```python
from build123d import *

# Parameters (mm, degrees)
EXTRUDE_1_DEPTH = 4
CHAMFER_1_SIZE  = 10


with BuildPart() as part:
    # Эскиз1 → Бобышка-Вытянуть1 (new, symmetric)
    with BuildSketch(Plane.XY):
        Polygon((0, 0), (0, 80), (8, 80), (70, 8), (70, 0), align=None)
    extrude(amount=EXTRUDE_1_DEPTH, both=True)

    # Фаска1
    chamfer_1_edges = [part.edges().sort_by_distance(p)[0] for p in [
        (0, 0, 0),
    ]]
    chamfer(chamfer_1_edges, length=CHAMFER_1_SIZE)


solid = part.part
```
Here's how the part is built. I have some questions about the finished solid (model axes, mm). Coordinates: 2 decimals unless noted, no trailing zeros. Loops run counter-clockwise (first coordinate to the right, second up) from the corner with the lowest first, then second, coordinate; pieces in that order, holes last. Notation, with made-up numbers: (11.25, -3) -> (31.25, -3) arc R21 cw to (31.25, 6) -> close; hole circle Ø8 at (-13, -12.5). An arc over 180 degrees is marked (long way). Return JSON: item names as keys, results as strings.
1) If we section it at C-C, the plane x = 45: Write out the boundary of the cut face in (y, z).
Results below:
{"outline": "(0, -4) -> (37.03, -4) -> (37.03, 4) -> (0, 4) -> close"}
2) If we section it at A-A, the plane z = -2: Write out the boundary of the cut face in (x, y).
Results below:
{"outline": "(0, 10) -> (10, 0) -> (70, 0) -> (70, 8) -> (8, 80) -> (0, 80) -> close"}
3) If we section it at B-B, the plane y = 41: Write out the boundary of the cut face in (x, z), then the cut area to 3 significant figures.
Results below:
{"outline": "(0, -4) -> (41.58, -4) -> (41.58, 4) -> (0, 4) -> close", "area": "333 mm²"}
4) I need wall thicknesses on line 1 (Y direction, x = 47.5, z = -0.5); line 2 (Y direction, x = 38.5, z = 3); line 3 (X direction, y = 23.5, z = 0.75). Which ranges of each line are inside material? Lowest first, please. Write a range as from..to.
Results below:
{"line 1": "0..34.13", "line 2": "0..44.58", "line 3": "0..56.65"}
